```python
from build123d import *

# Parameters (mm, degrees)
SKETCH1_R           = 15
BOSS_EXTRUDE1_DEPTH = 117
SKETCH2_R           = 15
BOSS_EXTRUDE2_DEPTH = 4
BOSS_EXTRUDE2_TAPER = 68
SKETCH3_R           = 5.099652586
BOSS_EXTRUDE3_DEPTH = 32
BOSS_EXTRUDE3_TAPER = 3.5
BOSS_EXTRUDE4_DEPTH = 3
SKETCH5_R           = 14
CUT_EXTRUDE1_DEPTH  = 117
SKETCH6_R           = 2.583886955
CUT_EXTRUDE2_DEPTH  = 117


with BuildPart() as part:
    # Sketch1 → Boss-Extrude1 (new body)
    with BuildSketch(Plane(origin=(0, 0, 0), x_dir=(0, 0, -1), z_dir=(1, 0, 0))):
        Circle(SKETCH1_R)
    extrude(amount=BOSS_EXTRUDE1_DEPTH)

    # Sketch2 → Boss-Extrude2 (add)
    with BuildSketch(Plane(origin=(117, 0, 0), x_dir=(0, 0, -1), z_dir=(1, 0, 0))):
        Circle(SKETCH2_R)
    extrude(amount=BOSS_EXTRUDE2_DEPTH, taper=BOSS_EXTRUDE2_TAPER)

    # Sketch3 → Boss-Extrude3 (add)
    with BuildSketch(Plane(origin=(121, 0, 0), x_dir=(0, 0, -1), z_dir=(1, 0, 0))):
        Circle(SKETCH3_R)
    extrude(amount=BOSS_EXTRUDE3_DEPTH, taper=BOSS_EXTRUDE3_TAPER)

    # Sketch4 → Boss-Extrude4 (add)
    with BuildSketch(Plane.ZY):
        with BuildLine():
            Line((9.96013089, -13.154739182), (26.54712441, -7.583677026))
            ThreePointArc((26.54712441, -7.583677026), (32, 0), (26.54712441, 7.583677026))
            Line((26.54712441, 7.583677026), (9.96013089, 13.154739182))
            ThreePointArc((9.96013089, 13.154739182), (0, 16.500041524), (-9.96013089, 13.154739182))
            Line((-9.96013089, 13.154739182), (-26.54712441, 7.583677026))
            ThreePointArc((-26.54712441, 7.583677026), (-32, 0), (-26.54712441, -7.583677026))
            Line((-26.54712441, -7.583677026), (-9.96013089, -13.154739182))
            ThreePointArc((-9.96013089, -13.154739182), (0, -16.500041524), (9.96013089, -13.154739182))
        make_face()
    extrude(amount=BOSS_EXTRUDE4_DEPTH)

    # Sketch5 → Cut-Extrude1 (cut)
    with BuildSketch(Plane.ZY.offset(3)):
        Circle(SKETCH5_R)
    extrude(amount=-CUT_EXTRUDE1_DEPTH, mode=Mode.SUBTRACT)

    # Sketch6 → Cut-Extrude2 (cut)
    with BuildSketch(Plane(origin=(153, 0, 0), x_dir=(0, 0, -1), z_dir=(1, 0, 0))):
        Circle(SKETCH6_R)
    extrude(amount=-CUT_EXTRUDE2_DEPTH, mode=Mode.SUBTRACT)


solid = part.part
```
Read the model definition and answer for the solid it produces. Units are mm, in the model's axes. A direction names the side the tool comes from. Round coordinates to 2 decimals unless told otherwise and drop trailing zeros. Write each loop counter-clockwise with the first axis right and the second up, starting at its lowest first coordinate (ties: lowest second). Pieces come first, ordered by that corner, then holes. Notation, with made-up numbers: M 71.25,47.25 L 105.25,47.25 A36 cw 105.25,86.25 Z; hole C 23,85.5 d5. An arc over 180 degrees is marked long. One line per item, written item: value.
Q1. Straight lines are drawn through the part: line 1 (Y direction, x = 34.5, z = 0); line 2 (Z direction, x = 145, y = 0.5); line 3 (X direction, y = -3, z = 25.5). For each, find the intervals that lie inside material, in ascending order. Write a range as [from, to].
Data:
line 1: [-15, -14], [14, 15]
line 2: [-3.6, -2.54], [2.54, 3.6]
line 3: [-3, 0]
Q2. Find section C-C on x = 134. Write down the section's boundary in (y, z), plus the area to 3 significant figures.
Data:
outline: C 0,0 d8.61; hole C 0,0 d5.17
area: 37.2 mm2
Q3. Find section A-A on z = 0. Write down the section's boundary in (x, y), plus the area to 3 significant figures.
Data:
outline: M -3,-16.5 L 0,-16.5 L 0,-15 L 117,-15 L 121,-5.1 L 153,-3.14 L 153,-2.58 L 114,-2.58 L 114,-14 L -3,-14 Z; M -3,14 L 114,14 L 114,2.58 L 153,2.58 L 153,3.14 L 121,5.1 L 117,15 L 0,15 L 0,16.5 L -3,16.5 Z
area: 476 mm2
Q4. Flat-ended cylindrical pins translate along their axes: pin 1 Ø2 at (y, z) = (-4, -8) entering from +X; pin 2 Ø3 at (x, y) = (76.5, -12.5) entering from -Z; pin 3 Ø8 at (x, z) = (50.5, -11.5) entering from +Y; pin 4 Ø12 at (x, z) = (31, -25.5) entering from +Y. Find the tip coordinate at first contact, or state that the pin passes through.
Data:
pin 1: x = 119.85
pin 2: z = -10.2
pin 3: y = 12.99
pin 4: through
Q5. For a pull along Z with two mould halves and no side action, classify faces 4 (the cylindrical face through (133.77, -1.57, 2.05)), 5 (the cylindrical face through (-1, 0, -32)), 6 (the flat face through (0, 5, -14.4)) as +Z half, -Z half, draft (parallel to the pull), parting line (faces both ways), or undercut.
Data:
face 4: undercut
face 5: -Z half
face 6: draft
Q6. Which of the six approach directions +Z, -Z, +X, -X, +Y, -Y give full straight-line access (tool end or side, diameter ignored) to faces 1 (the cylindrical face through (57.681, 0.66, 14.985)), 2 (the flat face through (114, 0, 3)), 3 (the flat face through (-1.479, 10.408, -18.138))?
Data:
face 1: +X
face 2: -X
face 3: -Z, +X, -X, +Y
Q7. Find section B-B on x = 71. Write down the section's boundary in (y, z), plus the area to 3 significant figures.
Data:
outline: C 0,0 d30; hole C 0,0 d28
area: 91.1 mm2
